Build history of the part. All positions in model axes, mm. Round coordinates to 2 decimals unless told otherwise and drop trailing zeros. Order: outer loops, then holes, each group sorted by start corner. A loop starts at its lowest first (then second) coordinate and runs counter-clockwise, first axis right, second up. Notation, with made-up numbers: (71.5, 26.5) -> (111.5, 26.5) arc R15 cw to (111.5, 31.5) -> close; hole circle Ø2 at (0.25, -22.75). An arc over 180 degrees is marked (long way). Answer as a JSON object with one key per item and string values.
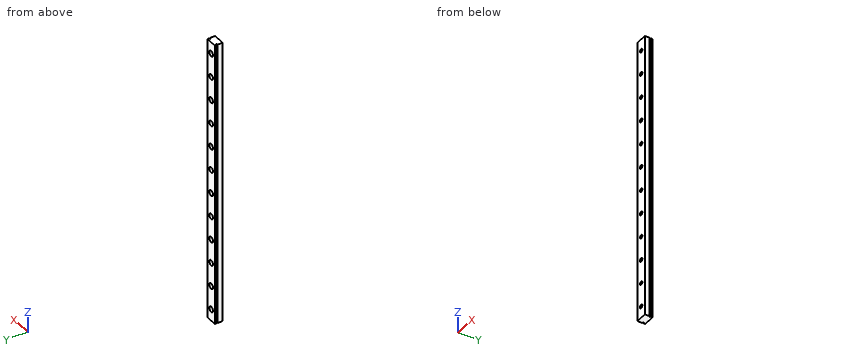
from build123d import *

# Parameters (mm, degrees)
BOSS_EXTRUDE1_DEPTH = 152.4
SKETCH2_R           = 2.921
CUT_EXTRUDE1_DEPTH  = 4.699
SKETCH4_R           = 1.905
CUT_EXTRUDE2_DEPTH  = 4.3782


with BuildPart() as part:
    # Sketch1 → Boss-Extrude1 (new body, symmetric)
    with BuildSketch(Plane.XY):
        with BuildLine():
            Line((-5.715, 2.0574), (-5.0419, 2.0574))
            ThreePointArc((-5.0419, 2.0574), (-4.862294878, 1.983005122), (-4.7879, 1.8034))
            Line((-4.7879, 1.8034), (-4.7879, 1.4732))
            ThreePointArc((-4.7879, 1.4732), (-4.862294878, 1.293594878), (-5.0419, 1.2192))
            Line((-5.0419, 1.2192), (-5.715, 1.2192))
            ThreePointArc((-5.715, 1.2192), (-5.894605122, 1.144805122), (-5.969, 0.9652))
            Line((-5.969, 0.9652), (-5.969, -3.7846))
            ThreePointArc((-5.969, -3.7846), (-5.894605122, -3.964205122), (-5.715, -4.0386))
            Line((-5.715, -4.0386), (5.715, -4.0386))
            ThreePointArc((5.715, -4.0386), (5.894605122, -3.964205122), (5.969, -3.7846))
            Line((5.969, -3.7846), (5.969, 0.9652))
            ThreePointArc((5.969, 0.9652), (5.894605122, 1.144805122), (5.715, 1.2192))
            Line((5.715, 1.2192), (5.0419, 1.2192))
            ThreePointArc((5.0419, 1.2192), (4.862294878, 1.293594878), (4.7879, 1.4732))
            Line((4.7879, 1.4732), (4.7879, 1.8034))
            ThreePointArc((4.7879, 1.8034), (4.862294878, 1.983005122), (5.0419, 2.0574))
            Line((5.0419, 2.0574), (5.715, 2.0574))
            ThreePointArc((5.715, 2.0574), (5.894605122, 2.131794878), (5.969, 2.3114))
            Line((5.969, 2.3114), (5.969, 3.7846))
            ThreePointArc((5.969, 3.7846), (5.894605122, 3.964205122), (5.715, 4.0386))
            Line((5.715, 4.0386), (-5.715, 4.0386))
            ThreePointArc((-5.715, 4.0386), (-5.894605122, 3.964205122), (-5.969, 3.7846))
            Line((-5.969, 3.7846), (-5.969, 2.3114))
            ThreePointArc((-5.969, 2.3114), (-5.894605122, 2.131794878), (-5.715, 2.0574))
        make_face()
    extrude(amount=BOSS_EXTRUDE1_DEPTH, both=True)

    # Sketch2 → Cut-Extrude1 (cut)
    with BuildSketch(Plane(origin=(0, 4.0386, 0), x_dir=(1, 0, 0), z_dir=(0, 1, 0))):
        with Locations((0, 139.954)):
            Circle(SKETCH2_R)
        with Locations((0, 114.507818182)):
            Circle(SKETCH2_R)
        with Locations((0, 89.061636364)):
            Circle(SKETCH2_R)
        with Locations((0, 63.615454545)):
            Circle(SKETCH2_R)
        with Locations((0, 38.169272727)):
            Circle(SKETCH2_R)
        with Locations((0, 12.723090909)):
            Circle(SKETCH2_R)
        with Locations((0, -12.723090909)):
            Circle(SKETCH2_R)
        with Locations((0, -38.169272727)):
            Circle(SKETCH2_R)
        with Locations((0, -63.615454545)):
            Circle(SKETCH2_R)
        with Locations((0, -89.061636364)):
            Circle(SKETCH2_R)
        with Locations((0, -114.507818182)):
            Circle(SKETCH2_R)
        with Locations((0, -139.954)):
            Circle(SKETCH2_R)
    extrude(amount=-CUT_EXTRUDE1_DEPTH, mode=Mode.SUBTRACT)

    # Sketch4 → Cut-Extrude2 (cut, through all)
    with BuildSketch(Plane(origin=(0, -0.6604, 0), x_dir=(1, 0, 0), z_dir=(0, 1, 0))):
        with Locations((0, 38.169272727)):
            Circle(SKETCH4_R)
        with Locations((0, 63.615454545)):
            Circle(SKETCH4_R)
        with Locations((0, 89.061636364)):
            Circle(SKETCH4_R)
        with Locations((0, 114.507818182)):
            Circle(SKETCH4_R)
        with Locations((0, 139.954)):
            Circle(SKETCH4_R)
        with Locations((0, -139.954)):
            Circle(SKETCH4_R)
        with Locations((0, -114.507818182)):
            Circle(SKETCH4_R)
        with Locations((0, -89.061636364)):
            Circle(SKETCH4_R)
        with Locations((0, -63.615454545)):
            Circle(SKETCH4_R)
        with Locations((0, -38.169272727)):
            Circle(SKETCH4_R)
        with Locations((0, -12.723090909)):
            Circle(SKETCH4_R)
        with Locations((0, 12.723090909)):
            Circle(SKETCH4_R)
    extrude(amount=-CUT_EXTRUDE2_DEPTH, mode=Mode.SUBTRACT)


solid = part.part
1) Cut at A-A, the plane y = -2.5. Count the separate pieces of the cut face and the enclosed holes in it, plus the area to 3 significant figures.
Checked values:
{"separate pieces": "1", "enclosed holes": "12", "area": "3,500 mm²"}
2) Flat gauge pins, fed straight in: pin 1 Ø1.8 at (x, z) = (0, 11.5) entering from +Y; pin 2 Ø3.5 at (x, z) = (0, -89.06) entering from -Y. Where does each tip first touch, or does it go through?
Checked values:
{"pin 1": "stops at y = -0.66", "pin 2": "passes through"}
3) Probe L1, parallel to Y at x = -5, z = 39; L2, parallel to X at y = 1, z = -20; L3, parallel to X at y = 1.5, z = 108. List the from-to ranges inside material, lowest first. Write a range as from..to.
Checked values:
{"L1": "y = -4.04..1.22, 2.05..4.04", "L2": "x = -5.97..5.97", "L3": "x = -4.79..4.79"}
4) Cut at B-B, the plane z = 2. Give the cut face in (x, y) (3 decimals).
Checked values:
{"outline": "(-5.969, -3.785) arc R0.254 ccw to (-5.715, -4.039) -> (5.715, -4.039) arc R0.254 ccw to (5.969, -3.785) -> (5.969, 0.965) arc R0.254 ccw to (5.715, 1.219) -> (5.042, 1.219) arc R0.254 cw to (4.788, 1.473) -> (4.788, 1.803) arc R0.254 cw to (5.042, 2.057) -> (5.715, 2.057) arc R0.254 ccw to (5.969, 2.311) -> (5.969, 3.785) arc R0.254 ccw to (5.715, 4.039) -> (-5.715, 4.039) arc R0.254 ccw to (-5.969, 3.785) -> (-5.969, 2.311) arc R0.254 ccw to (-5.715, 2.057) -> (-5.042, 2.057) arc R0.254 cw to (-4.788, 1.803) -> (-4.788, 1.473) arc R0.254 cw to (-5.042, 1.219) -> (-5.715, 1.219) arc R0.254 ccw to (-5.969, 0.965) -> close"}
